from build123d import *


with BuildPart() as part:
    # Sketch1 → Revolve1 (revolve)
    with BuildSketch(Plane.XY):
        with BuildLine():
            Line((0, 22), (0, 0))
            Line((0, 0), (17.5, 0))
            Line((17.5, 0), (17.5, -3))
            Line((17.5, -3), (20.5, -3))
            Line((20.5, -3), (20.5, 0))
            Line((20.5, 0), (25, 0))
            ThreePointArc((25, 0), (16.747123528, 4.115577986), (7.849471791, 6.540396696))
            ThreePointArc((7.849471791, 6.540396696), (5.599395212, 8.301845982), (5.845351334, 11.148783597))
            ThreePointArc((5.845351334, 11.148783597), (6.162731327, 18.319750381), (0, 22))
        make_face()
    revolve(axis=Axis((0, 0, 0), (0, 1, 0)))


solid = part.part
Could you check a few things on this model? Use its own coordinates, in mm. Coordinates: 2 decimals unless noted, no trailing zeros. Write each loop counter-clockwise with the first axis right and the second up, starting at its lowest first coordinate (ties: lowest second). Pieces come first, ordered by that corner, then holes. Notation, with made-up numbers: M -5.5,7.5 L 25.5,7.5 A20 ccw 25.5,38.5 Z; hole C -2,5 d8. An arc over 180 degrees is marked long. One line per question, with ' | ' between items.
1) Imagine slicing it at B-B, the plane z = -12. Write out the boundary of the cut face in (x, y), and give its area (3 significant figures).
Checks:
outline: M -21.93,0 L -16.62,0 L -16.62,-3 L -12.74,-3 L -12.74,0 L 12.74,0 L 12.74,-3 L 16.62,-3 L 16.62,0 L 21.93,0 A45.44 ccw Z | area: 190 mm²
2) I need wall thicknesses on probe 1 along Z at (x, y) = (0, -1.45); probe 2 along Y at (x, z) = (6, 4). Which ranges of each line are inside material? Lowest first, please. Write a range as [from, to].
Checks:
probe 1: [-20.5, -17.5], [17.5, 20.5] | probe 2: [0, 6.72]
3) Imagine slicing it at A-A, the plane x = -12. Write out the boundary of the cut face in (y, z), and give its area (3 significant figures).
Checks:
outline: M -3,-16.62 L 0,-16.62 L 0,-21.93 A45.44 ccw 0,21.93 L 0,16.62 L -3,16.62 L -3,12.74 L 0,12.74 L 0,-12.74 L -3,-12.74 Z | area: 190 mm²
4) Imagine slicing it at D-D, the plane z = 0. Write out the boundary of the cut face in (x, y), and give its area (3 significant figures).
Checks:
outline: M -25,0 L -20.5,0 L -20.5,-3 L -17.5,-3 L -17.5,0 L 17.5,0 L 17.5,-3 L 20.5,-3 L 20.5,0 L 25,0 A47 ccw 7.85,6.54 A3 cw 5.85,11.15 A7 ccw long -5.85,11.15 A3 cw -7.85,6.54 A47 ccw Z | area: 437 mm²
5) For pin 1 Ø1 at (y, z) = (13, 5.5) entering from +X; pin 2 Ø5 at (x, z) = (-0.5, -3.5) entering from +Y; pin 3 Ø10 at (y, z) = (8.5, 3) entering from +X, each with a flat end and sliding along its axis, tell me the tip position at first contact or that it passes through.
Checks:
pin 1: x = 4.51 | pin 2: y = 21.92 | pin 3: x = 18.06
6) Imagine slicing it at C-C, the plane y = 13.25. Write out the boundary of the cut face in (x, z).
Checks:
outline: C 0,0 d13.56
7) If we mould it in two halves opening along Z, with no side actions, what happens to faces 1 (the face through (3.8, 0, -20.5)), 2 (the face through (0, 0, 0)), 3 (the face through (-13.887, -1.521, 10.648)), 4 (the face through (-4.444, -1.479, 20.013))? For each: released by +Z, released by -Z, zero draft, split by the parting line, or undercut.
Checks:
face 1: zero draft | face 2: undercut | face 3: undercut | face 4: split by the parting line
